CAD build for the part. Positions are in the model's coordinates, mm. Face numbers are marked on the shaded views. A direction names the side the tool comes from. Round coordinates to 2 decimals unless told otherwise and drop trailing zeros. Order: outer loops, then holes, each group sorted by start corner. A loop starts at its lowest first (then second) coordinate and runs counter-clockwise, first axis right, second up.
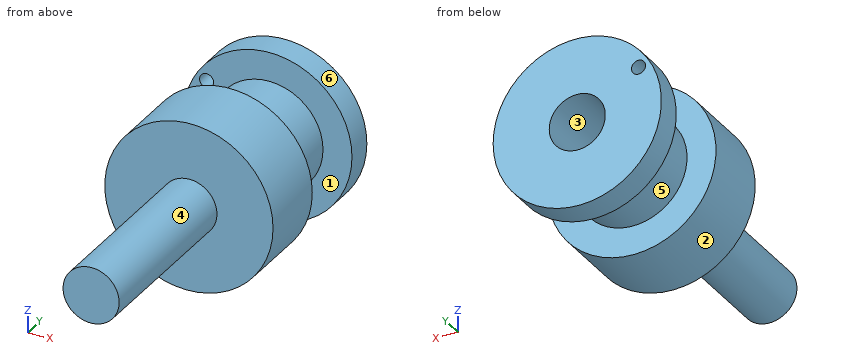
```python
from build123d import *

# Parameters (mm, degrees)
SKETCH1_R           = 3
BOSS_EXTRUDE1_DEPTH = 19.7
SKETCH2_R           = 9
BOSS_EXTRUDE2_DEPTH = 7.9
SKETCH3_R           = 5.9
BOSS_EXTRUDE3_DEPTH = 8
SKETCH4_R           = 9
BOSS_EXTRUDE4_DEPTH = 3
SKETCH5_R           = 3
CUT_EXTRUDE1_DEPTH  = 9.6
SKETCH7_R           = 0.75
CUT_EXTRUDE2_DEPTH  = 10


with BuildPart() as part:
    # Sketch1 → Boss-Extrude1 (new body)
    with BuildSketch(Plane(origin=(0, 0, 0), x_dir=(1, 0, 0), z_dir=(0, 1, 0))):
        Circle(SKETCH1_R)
    extrude(amount=BOSS_EXTRUDE1_DEPTH)

    # Sketch2 → Boss-Extrude2 (add)
    with BuildSketch(Plane(origin=(0, 19.7, 0), x_dir=(1, 0, 0), z_dir=(0, 1, 0))):
        Circle(SKETCH2_R)
    extrude(amount=BOSS_EXTRUDE2_DEPTH)

    # Sketch3 → Boss-Extrude3 (add)
    with BuildSketch(Plane(origin=(0, 27.6, 0), x_dir=(1, 0, 0), z_dir=(0, 1, 0))):
        Circle(SKETCH3_R)
    extrude(amount=BOSS_EXTRUDE3_DEPTH)

    # Sketch4 → Boss-Extrude4 (add)
    with BuildSketch(Plane(origin=(0, 35.6, 0), x_dir=(1, 0, 0), z_dir=(0, 1, 0))):
        Circle(SKETCH4_R)
    extrude(amount=BOSS_EXTRUDE4_DEPTH)

    # Sketch5 → Cut-Extrude1 (cut)
    with BuildSketch(Plane(origin=(0, 38.6, 0), x_dir=(1, 0, 0), z_dir=(0, 1, 0))):
        Circle(SKETCH5_R)
    extrude(amount=-CUT_EXTRUDE1_DEPTH, mode=Mode.SUBTRACT)

    # Sketch7 → Cut-Extrude2 (cut)
    with BuildSketch(Plane(origin=(0, 38.6, 0), x_dir=(1, 0, 0), z_dir=(0, 1, 0))):
        with Locations((-6.55100535, -4.239956241)):
            Circle(SKETCH7_R)
    extrude(amount=-CUT_EXTRUDE2_DEPTH, mode=Mode.SUBTRACT)


solid = part.part
```
1. Drill centre lines: line 1 (X direction, y = 31.5, z = 0); line 2 (Y direction, x = 5, z = -6.25); line 3 (Y direction, x = -1.75, z = 0). Where is each one in solid material? Low to high.
2. Cut at D-D, the plane x = 0. Write the cut outline in (y, z), and give its area (3 significant figures).
3. Pin check, flat tips, straight feed: P1, Ø1.2, axis at x = -6.55, z = 4.24, coming from the +Y side; P2, Ø2, axis at x = 1, z = -5.5, coming from the -Y side; P3, Ø2, axis at x = -6, y = 33.5, coming from the +Z side. Stop position of each tip, or through.
4. Cut at B-B, the plane x = 7.5. Write the cut outline in (y, z), and give its area (3 significant figures).
5. Tool access for the marked faces 4, 5 and 6: list every direction of +Z, -Z, +X, -X, +Y, -Y with a clear straight run to the whole face (end or side of a thin tool).
6. Cut at A-A, the plane z = 0. Write the cut outline in (x, y), and give its area (3 significant figures).
7. Mould opens along X. For the marked faces 1, 2 and 3 say: released by +X, released by -X, zero draft, split by the parting line, or undercut.
8. Cut at C-C, the plane y = 34. Write the cut outline in (x, z), and give its area (3 significant figures).
Outcome:
1. line 1: x = -5.9 to -3, 3 to 5.9
1. line 2: y = 19.7 to 27.6, 35.6 to 38.6
1. line 3: y = 0 to 29
2. outline: (0, -3) - (19.7, -3) - (19.7, -9) - (27.6, -9) - (27.6, -5.9) - (35.6, -5.9) - (35.6, -9) - (38.6, -9) - (38.6, -3) - (29, -3) - (29, 3) - (38.6, 3) - (38.6, 9) - (35.6, 9) - (35.6, 5.9) - (27.6, 5.9) - (27.6, 9) - (19.7, 9) - (19.7, 3) - (0, 3) - close
2. area: 351 mm2
3. P1: stops at y = 27.6
3. P2: stops at y = 19.7
3. P3: stops at z = 3.13
4. outline: (19.7, -4.97) - (27.6, -4.97) - (27.6, 4.97) - (19.7, 4.97) - close; (35.6, -4.97) - (38.6, -4.97) - (38.6, 4.97) - (35.6, 4.97) - close
4. area: 108 mm2
5. face 4: -Y
5. face 5: none
5. face 6: +Y, -Y
6. outline: (-9, 19.7) - (-3, 19.7) - (-3, 0) - (3, 0) - (3, 19.7) - (9, 19.7) - (9, 27.6) - (5.9, 27.6) - (5.9, 35.6) - (9, 35.6) - (9, 38.6) - (3, 38.6) - (3, 29) - (-3, 29) - (-3, 38.6) - (-9, 38.6) - (-9, 35.6) - (-5.9, 35.6) - (-5.9, 27.6) - (-9, 27.6) - close
6. area: 351 mm2
7. face 1: zero draft
7. face 2: split by the parting line
7. face 3: undercut
8. outline: circle Ø11.8 at (0, 0); hole circle Ø6 at (0, 0)
8. area: 81.1 mm2
